Geometry check sheet. Reference: drawing and pictorial views, mm from the part's lowest x, y, z. Coordinates: 2 decimals unless noted, no trailing zeros. Write each loop counter-clockwise with the first axis right and the second up, starting at its lowest first coordinate (ties: lowest second). Pieces come first, ordered by that corner, then holes. Notation, with made-up numbers: (45.25, 60) -> (57.25, 60) arc R20 cw to (57.25, 75) -> close; hole circle Ø10 at (36, -6.5). An arc over 180 degrees is marked (long way). Answer in a Markdown table with one row per item.
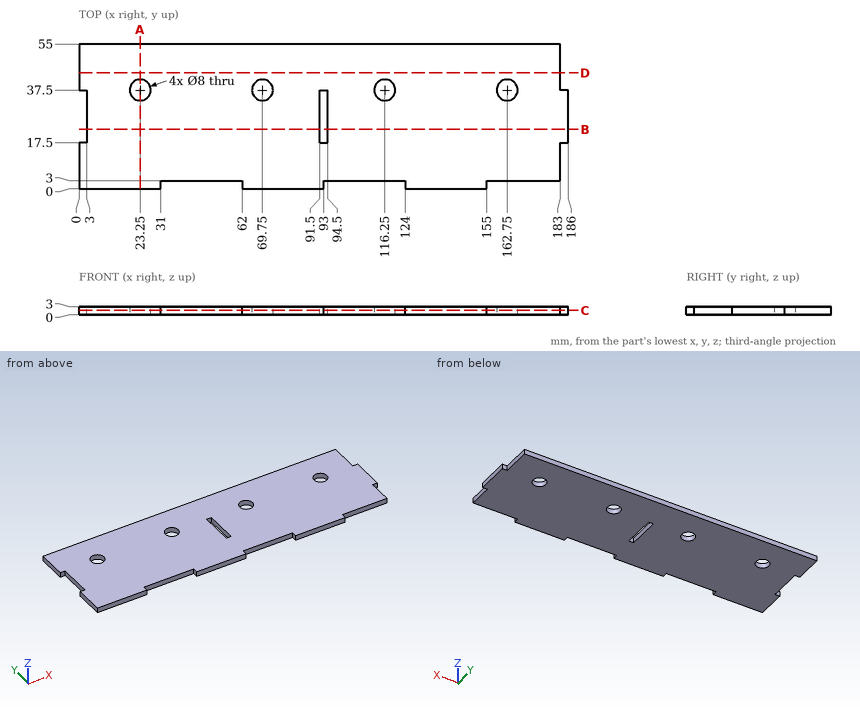
1. Section check D-D, the plane y = 44. Record the boundary of the cut face in (x, z), plus the area to 3 significant figures.
Geometry says:
| item | result |
|---|---|
| outline | (0, 0) -> (183, 0) -> (183, 3) -> (0, 3) -> close |
| area | 549 mm^2 |
2. Section check A-A, the plane x = 23.25. Record the boundary of the cut face in (y, z), plus the area to 3 significant figures.
Geometry says:
| item | result |
|---|---|
| outline | (0, 0) -> (33.5, 0) -> (33.5, 3) -> (0, 3) -> close; (41.5, 0) -> (55, 0) -> (55, 3) -> (41.5, 3) -> close |
| area | 141 mm^2 |
3. Depth check by flat-ended pin: P1, Ø13, axis at x = 69.75, y = 37.5, coming from the +Z side; P2, Ø1.5, axis at x = 107.5, z = 1.5, coming from the -Y side; P3, Ø0.9, axis at y = 48, z = 1.5, coming from the +X side; P4, Ø0.9, axis at y = 28.5, z = 1, coming from the -X side. Enter the tip coordinate at first touch or a pass-through.
Geometry says:
| item | result |
|---|---|
| P1 | z = 3 |
| P2 | y = 3 |
| P3 | x = 183 |
| P4 | x = 3 |
4. Section check B-B, the plane y = 22.5. Record the boundary of the cut face in (x, z), plus the area to 3 significant figures.
Geometry says:
| item | result |
|---|---|
| outline | (3, 0) -> (91.5, 0) -> (91.5, 3) -> (3, 3) -> close; (94.5, 0) -> (186, 0) -> (186, 3) -> (94.5, 3) -> close |
| area | 540 mm^2 |
5. Section check C-C, the plane z = 1.6. State how many separate pieces and enclosed holes the cut face has, plus the area to 3 significant figures.
Geometry says:
| item | result |
|---|---|
| separate pieces | 1 |
| enclosed holes | 5 |
| area | 9,530 mm^2 |
6. Thickness scan on line 1 (Y direction, x = 69.75, z = 0.85); line 2 (X direction, y = 31, z = 1.9); line 3 (Y direction, x = 162.75, z = 1.75). Record the ranges inside material, lowest first. Write a range as from..to.
Geometry says:
| item | result |
|---|---|
| line 1 | 0..33.5, 41.5..55 |
| line 2 | 3..91.5, 94.5..186 |
| line 3 | 3..33.5, 41.5..55 |
